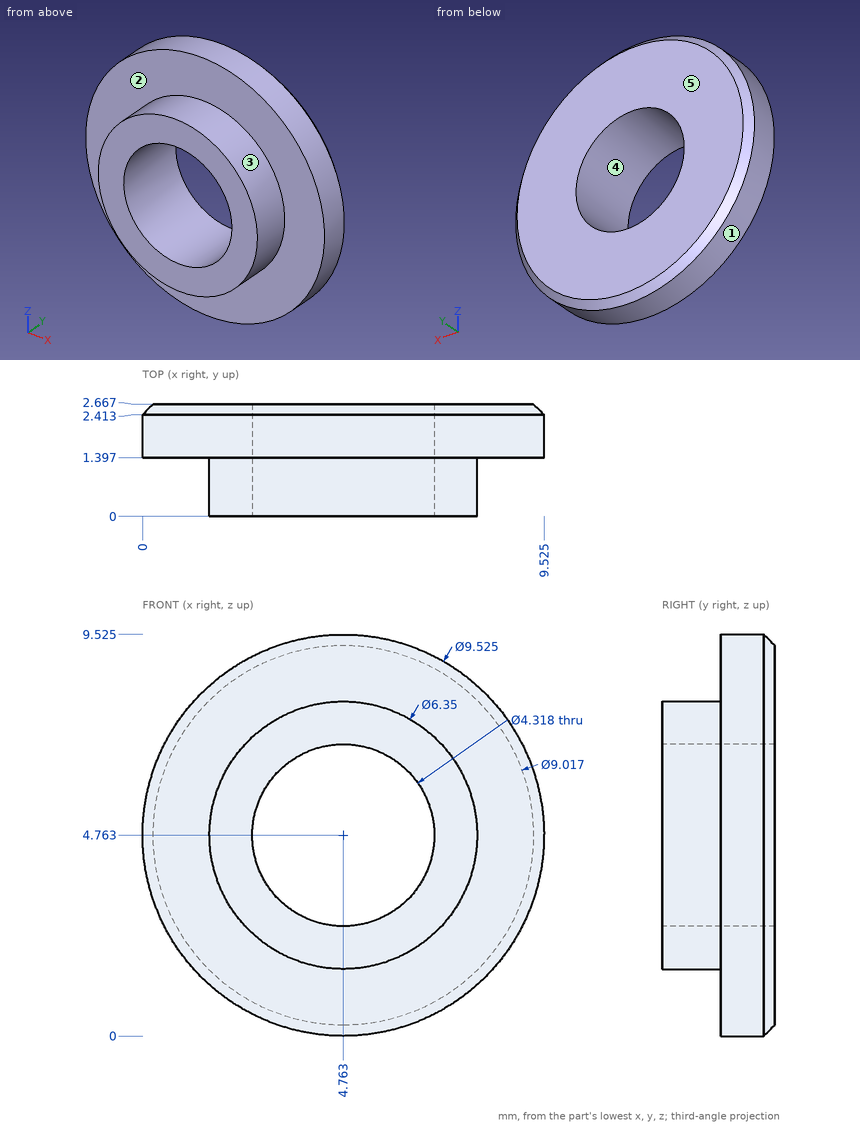
Part print with two shaded views. Sizes in mm from the minimum x, y, z corner. A direction names the side the tool comes from. Coordinates: 2 decimals unless noted, no trailing zeros.
(1) Pin check, flat tips, straight feed: pin 1 Ø5 at (x, z) = (4.5, 6.5) entering from -Y; pin 2 Ø1.5 at (x, z) = (4, 5) entering from -Y. Stop position of each tip, or through.
Solution:
pin 1: stops at y = 0
pin 2: passes through
(2) Drill centre lines: L1, parallel to X at y = 1.45, z = 4.75 (1 decimal); L2, parallel to Y at x = 6.25, z = 8.25; L3, parallel to Z at x = 4.5, y = 0.9 (1 decimal). Where is each one in solid material? Low to high.
Solution:
L1: x = 0 to 2.6, 6.9 to 9.5
L2: y = 1.4 to 2.67
L3: z = 1.6 to 2.6, 6.9 to 7.9
(3) Mould opens along Z. For the marked faces 3, 4 and 5 say: released by +Z, released by -Z, zero draft, split by the parting line, or undercut.
Solution:
face 3: split by the parting line
face 4: undercut
face 5: zero draft
(4) Which spindle directions (+Z, -Z, +X, -X, +Y, -Y) get a long thin tool onto all of the face, cutting with end or side? Do the marked faces 1 and 2. Say none if no direction does.
Solution:
face 1: +Y, -Y
face 2: -Y
